The figure shows three views and two pictorial views of one solid part (mm, origin at its lowest corner). Answer the questions. A direction names the side the tool comes from. Round coordinates to 2 decimals unless told otherwise and drop trailing zeros. Write each loop counter-clockwise with the first axis right and the second up, starting at its lowest first coordinate (ties: lowest second). Pieces come first, ordered by that corner, then holes. Notation, with made-up numbers: M 76.5,31.25 L 135.5,31.25 A23 ccw 135.5,47.25 Z; hole C -38,56.25 d2. An arc over 180 degrees is marked long. Answer in a Markdown table with one row per item.
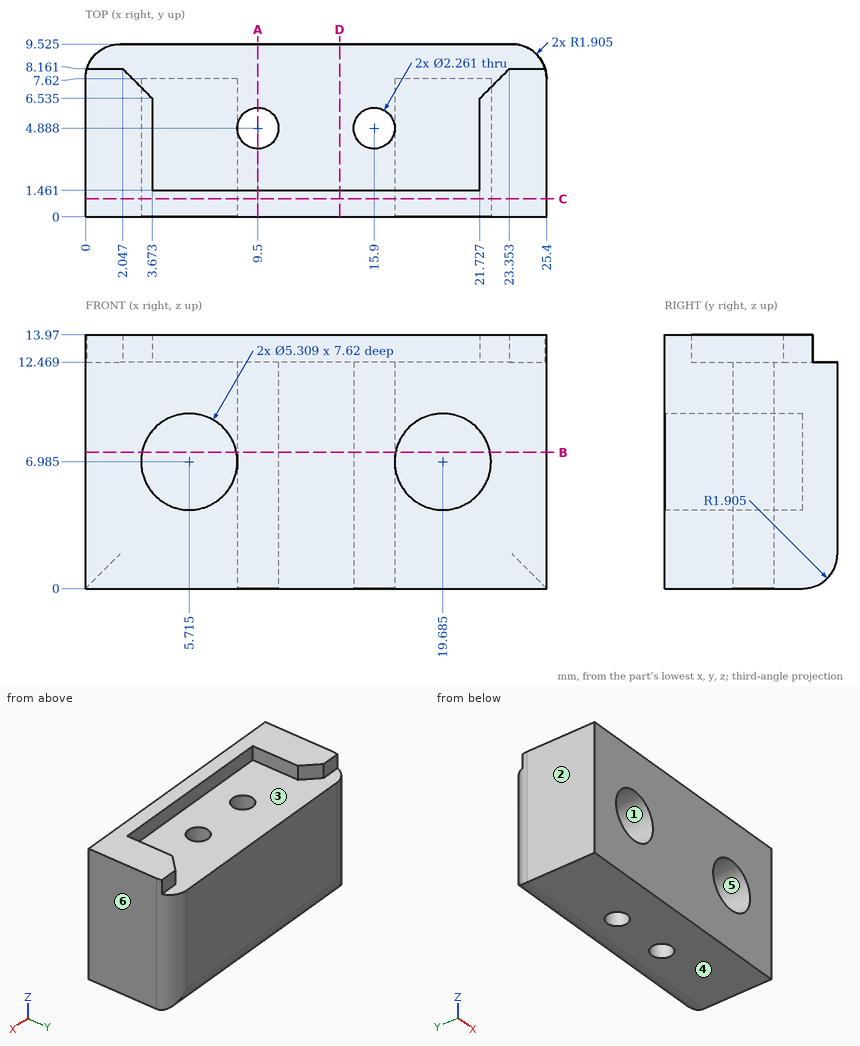
1. Given pin 1 (3 mm diameter, centred on x = 12.5, z = 4.5, fed in from -Y); pin 2 (1.2 mm diameter, centred on x = 16.5, z = 13.5, fed in from +Y); pin 3 (3 mm diameter, centred on x = 5.715, z = 6.985, fed in from -Y); pin 4 (2.5 mm diameter, centred on x = 19, y = 5, fed in from +Z), each flat-ended and moving along its own axis, determine where each tip first touches the part or whether it passes through.
Calculated:
| item | result |
|---|---|
| pin 1 | stops at y = 0 |
| pin 2 | stops at y = 1.46 |
| pin 3 | stops at y = 7.62 |
| pin 4 | stops at z = 12.47 |
2. The part is cut by section C-C (y = 1). Determine the outline of the cut face in (x, z) (1 decimal).
Calculated:
| item | result |
|---|---|
| outline | M 0,0 L 25.4,0 L 25.4,14 L 0,14 Z; hole C 5.7,7 d5.3; hole C 19.7,7 d5.3 |
3. A tool of negligible diameter and unlimited length cuts with its end or side. For the marked faces 1, 2 and 3, from which of +Z, -Z, +X, -X, +Y, -Y can it reach the whole face along a straight path? Write none if from no direction.
Calculated:
| item | result |
|---|---|
| face 1 | -Y |
| face 2 | +Z, -Z, -X, +Y, -Y |
| face 3 | +Z, +Y |
4. The part is cut by section D-D (x = 14). Determine the outline of the cut face in (y, z) (1 decimal).
Calculated:
| item | result |
|---|---|
| outline | M 0,0 L 7.6,0 A1.9 ccw 9.5,1.9 L 9.5,12.5 L 1.5,12.5 L 1.5,14 L 0,14 Z |
5. Consider line 1 along Y through (x, z) = (15.9, 6.25) (1 decimal); line 2 along Z through (x, y) = (19.75, 3.25); line 3 along X through (y, z) = (5.25, 2). Determine where each line is inside the solid, lowest interval first. Write a range as from..to.
Calculated:
| item | result |
|---|---|
| line 1 | y = 0..3.8, 6..9.5 |
| line 2 | z = 0..4.33, 9.64..12.47 |
| line 3 | x = 0..8.43, 10.57..14.83, 16.97..25.4 |
6. The part is cut by section A-A (x = 9.5). Determine the outline of the cut face in (y, z) (1 decimal).
Calculated:
| item | result |
|---|---|
| outline | M 0,0 L 3.8,0 L 3.8,12.5 L 1.5,12.5 L 1.5,14 L 0,14 Z; M 6,0 L 7.6,0 A1.9 ccw 9.5,1.9 L 9.5,12.5 L 6,12.5 Z |
7. The part is cut by section B-B (z = 7.5). Determine the outline of the cut face in (x, y) (1 decimal), plus the area to 3 significant figures.
Calculated:
| item | result |
|---|---|
| outline | M 0,0 L 3.1,0 L 3.1,7.6 L 8.3,7.6 L 8.3,0 L 17.1,0 L 17.1,7.6 L 22.3,7.6 L 22.3,0 L 25.4,0 L 25.4,7.6 A1.9 ccw 23.5,9.5 L 1.9,9.5 A1.9 ccw 0,7.6 Z; hole C 9.5,4.9 d2.3; hole C 15.9,4.9 d2.3 |
| area | 153 mm² |
8. Determine the mould class of the marked faces 4, 5 and 6 for opening direction Z: released by +Z, released by -Z, zero draft, split by the parting line, or undercut.
Calculated:
| item | result |
|---|---|
| face 4 | released by -Z |
| face 5 | undercut |
| face 6 | zero draft |
